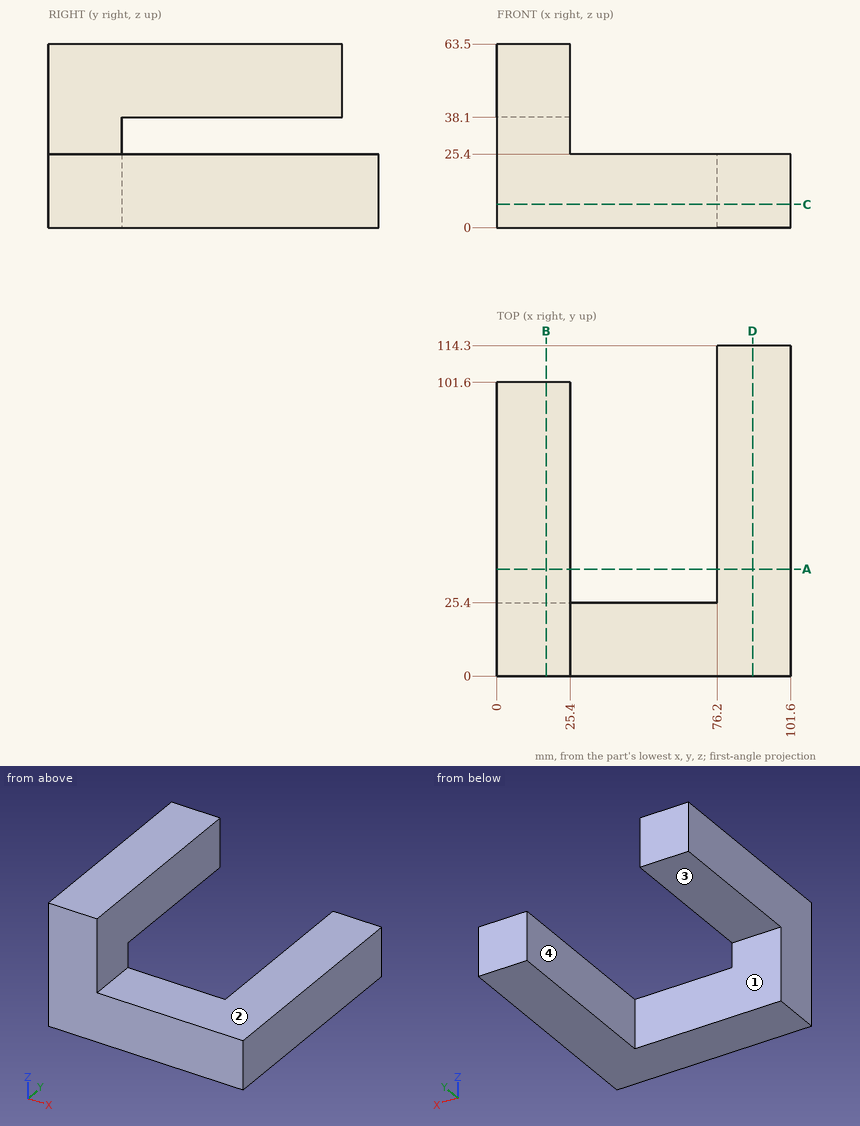
Here's the drawing with two shaded views (mm, measured from the low corner). I have some questions. A direction names the side the tool comes from. Round coordinates to 2 decimals unless told otherwise and drop trailing zeros. Loops run counter-clockwise (first coordinate to the right, second up) from the corner with the lowest first, then second, coordinate; pieces in that order, holes last. Notation, with made-up numbers: (65.25, 58) -> (105.25, 58) arc R13 ccw to (105.25, 65) -> close; hole circle Ø1 at (-17.75, 22). An arc over 180 degrees is marked (long way). Answer as CSV lines item,"result". Start each with the question number.
1. For the marked faces 1, 2, 3 and 4, which set-ups out of +Z, -Z, +X, -X, +Y, -Y let a thin tool reach every point of the face, with its end or its side?
2. I'm going to push flat-ended pins straight in: P1, Ø23, axis at x = 62.5, y = 81.5, coming from the +Z side; P2, Ø20.5, axis at y = 62, z = 17, coming from the -X side; P3, Ø20.5, axis at x = 17.5, z = 45, coming from the +Y side; P4, Ø8, axis at x = 57.5, z = 9.5, coming from the -Y side. Where does each tip first touch, or does it pass through?
3. Imagine slicing it at C-C on z = 8. Write out the boundary of the cut face in (x, y), plus the area to 3 significant figures.
4. I need wall thicknesses on probe 1 along Y at (x, z) = (46, 17.5); probe 2 along X at (y, z) = (51, 19). Which ranges of each line are inside material? Lowest first, please. Write a range as from..to.
5. Imagine slicing it at D-D on x = 88.5. Write out the boundary of the cut face in (y, z).
6. Imagine slicing it at B-B on x = 17. Write out the boundary of the cut face in (y, z).
7. Imagine slicing it at A-A on y = 37. Write out the boundary of the cut face in (x, z), plus the area to 3 significant figures.
Solution:
1,face 1,"-Z, -X, +Y"
1,face 2,"+Z, +X, +Y, -Y"
1,face 3,"-Z, +X, -X, +Y"
1,face 4,"+Z, -Z, -X, +Y"
2,P1,"through"
2,P2,"x = 76.2"
2,P3,"y = 101.6"
2,P4,"y = 0"
3,outline,"(0, 0) -> (101.6, 0) -> (101.6, 114.3) -> (76.2, 114.3) -> (76.2, 25.4) -> (0, 25.4) -> close"
3,area,"4,840 mm²"
4,probe 1,"0..25.4"
4,probe 2,"76.2..101.6"
5,outline,"(0, 0) -> (114.3, 0) -> (114.3, 25.4) -> (0, 25.4) -> close"
6,outline,"(0, 0) -> (25.4, 0) -> (25.4, 38.1) -> (101.6, 38.1) -> (101.6, 63.5) -> (0, 63.5) -> close"
7,outline,"(0, 38.1) -> (25.4, 38.1) -> (25.4, 63.5) -> (0, 63.5) -> close; (76.2, 0) -> (101.6, 0) -> (101.6, 25.4) -> (76.2, 25.4) -> close"
7,area,"1,290 mm²"
